from build123d import *

# Parameters (mm, degrees)
SKETCH1_W           = 6
SKETCH1_H           = 9
SKETCH1_W_2         = 20
SKETCH1_H_2         = 15.579203612
BOSS_EXTRUDE1_DEPTH = 6


with BuildPart() as part:
    # Sketch1 → Boss-Extrude1 (new body)
    with BuildSketch(Plane(origin=(0, 0, 0), x_dir=(1, 0, 0), z_dir=(0, 1, 0))):
        Polygon((-27.97781142, 17.579932433), (-27.97781142, -16.909955783), (12.733891313, -16.909955783), (12.733891313, 17.579932433), (12.733891313, 38.430995495), (12.733891313, 47.430995495), (8.378039947, 47.430995495), (8.378039947, 38.430995495), (-23.621960053, 38.430995495), (-23.621960053, 47.430995495), (-27.97781142, 47.430995495), (-27.97781142, 38.430995495), align=None)
        with Locations((5.378039947, 8.930995495)):
            Rectangle(SKETCH1_W, SKETCH1_H, mode=Mode.SUBTRACT)
        with Locations((5.378039947, -10.069004505)):
            Rectangle(SKETCH1_W, SKETCH1_H, mode=Mode.SUBTRACT)
        with Locations((-20.621960053, 8.930995495)):
            Rectangle(SKETCH1_W, SKETCH1_H, mode=Mode.SUBTRACT)
        with Locations((-20.621960053, -10.069004505)):
            Rectangle(SKETCH1_W, SKETCH1_H, mode=Mode.SUBTRACT)
        with Locations((-7.621960053, 24.641393689)):
            Rectangle(SKETCH1_W_2, SKETCH1_H_2, mode=Mode.SUBTRACT)
    extrude(amount=BOSS_EXTRUDE1_DEPTH)


solid = part.part
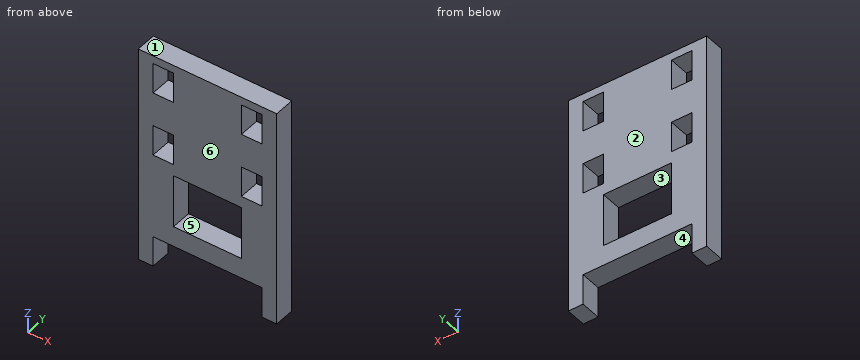
Work out the finished part from the listing and answer in its coordinate system (mm). Face numbers are marked on the shaded views. A direction names the side the tool comes from. Round coordinates to 2 decimals unless told otherwise and drop trailing zeros. Loops run counter-clockwise (first coordinate to the right, second up) from the corner with the lowest first, then second, coordinate; pieces in that order, holes last. Notation, with made-up numbers: (62, 4) - (110, 4) arc R23 cw to (110, 27) - close; hole circle Ø2 at (6, 51). An arc over 180 degrees is marked (long way). Use one line per item in the form item = value. Start each with the question number.
(1) Find section A-A on x = 0.5. Determine the outline of the cut face in (y, z).
(2) Consider line 1 (Z direction, x = -22, y = 5.15); line 2 (X direction, y = 1, z = 12); line 3 (Z direction, x = -11, y = 0.5). Determine where each line is inside the solid, lowest interval first.
(3) Which of the six approach directions +Z, -Z, +X, -X, +Y, -Y give full straight-line access (tool end or side, diameter ignored) to the marked faces 4, 5 and 6?
(4) A flat-ended cylindrical pin translates along its axis: P1, Ø3, axis at x = -8.5, y = 3, coming from the -Z side. Find the tip coordinate at first contact, or state that the pin passes through.
(5) Find section B-B on z = -43. Determine the outline of the cut face in (x, y), and give its area (3 significant figures).
(6) Find section D-D on z = -10.5. Determine the outline of the cut face in (x, y), and give its area (3 significant figures).
(7) Find section C-C on y = 5.05. Determine the outline of the cut face in (x, z).
(8) Determine the mould class of the marked faces 1, 2 and 3 for opening direction Z: +Z half, -Z half, draft (parallel to the pull), parting line (faces both ways), or undercut.
Answer list:
q1.outline = (0, -38.43) - (6, -38.43) - (6, -32.43) - (0, -32.43) - close; (0, -16.85) - (6, -16.85) - (6, 16.91) - (0, 16.91) - close
q2.line_1 = -38.43 to -13.43, -4.43 to 5.57, 14.57 to 16.91
q2.line_2 = -27.98 to -23.62, -17.62 to 2.38, 8.38 to 12.73
q2.line_3 = -38.43 to -32.43, -16.85 to 16.91
q3.face_4 = -Z, +Y, -Y
q3.face_5 = +Y, -Y
q3.face_6 = +Z, -Z, +X, -X, -Y
q4.P1 = -38.43
q5.outline = (-27.98, 0) - (-23.62, 0) - (-23.62, 6) - (-27.98, 6) - close; (8.38, 0) - (12.73, 0) - (12.73, 6) - (8.38, 6) - close
q5.area = 52.3 mm^2
q6.outline = (-27.98, 0) - (-23.62, 0) - (-23.62, 6) - (-27.98, 6) - close; (-17.62, 0) - (2.38, 0) - (2.38, 6) - (-17.62, 6) - close; (8.38, 0) - (12.73, 0) - (12.73, 6) - (8.38, 6) - close
q6.area = 172 mm^2
q7.outline = (-27.98, -47.43) - (-23.62, -47.43) - (-23.62, -38.43) - (8.38, -38.43) - (8.38, -47.43) - (12.73, -47.43) - (12.73, 16.91) - (-27.98, 16.91) - close; hole (-23.62, -13.43) - (-17.62, -13.43) - (-17.62, -4.43) - (-23.62, -4.43) - close; hole (-23.62, 5.57) - (-17.62, 5.57) - (-17.62, 14.57) - (-23.62, 14.57) - close; hole (-17.62, -32.43) - (2.38, -32.43) - (2.38, -16.85) - (-17.62, -16.85) - close; hole (2.38, -13.43) - (8.38, -13.43) - (8.38, -4.43) - (2.38, -4.43) - close; hole (2.38, 5.57) - (8.38, 5.57) - (8.38, 14.57) - (2.38, 14.57) - close
q8.face_1 = +Z half
q8.face_2 = draft
q8.face_3 = undercut
